The drawing under review shows one solid part. Ordinate dimensions are in mm from its lowest x, y, z. Coordinates: 2 decimals unless noted, no trailing zeros. Loops run counter-clockwise (first coordinate to the right, second up) from the corner with the lowest first, then second, coordinate; pieces in that order, holes last. Notation, with made-up numbers: (-20.75, 51.5) - (14.25, 51.5) arc R14 ccw to (14.25, 56.5) - close; hole circle Ø1 at (65.5, 43). An arc over 180 degrees is marked (long way). Answer as a JSON object with one key per item and string values. Group by question number.
Item 1: Mouldability with a two-part tool opening along Y and no side actions: class the marked faces 1, 2 and 3 as released by +Y, released by -Y, zero draft, split by the parting line, or undercut.
Item 2: Clearance check with flat-ended pins moving along their axes: pin 1 (6 mm diameter, centred on x = 5.5, y = 25, fed in from -Z); pin 2 (3 mm diameter, centred on y = 2.51, z = 2.5, fed in from -X); pin 3 (2 mm diameter, centred on y = 2.51, z = 2.5, fed in from -X). State where each tip first meets the part, or that it passes through.
Item 3: We need section D-D (y = 17). Give the boundary of the cut face in (x, z), then the cut area to 3 significant figures.
Item 4: We need section B-B (y = 13). Give the boundary of the cut face in (x, z).
Item 5: To check wall thickness, follow line 1 (X direction, y = 4.5, z = 4.55); line 2 (Y direction, x = 15.5, z = 1.55) (1 decimal); line 3 (X direction, y = 13, z = 3.5). State the ranges of each line that lie inside material, in increasing order.
Item 6: We need section C-C (x = 8.25). Give the boundary of the cut face in (y, z).
Item 7: We need section A-A (x = 16). Give the boundary of the cut face in (y, z).
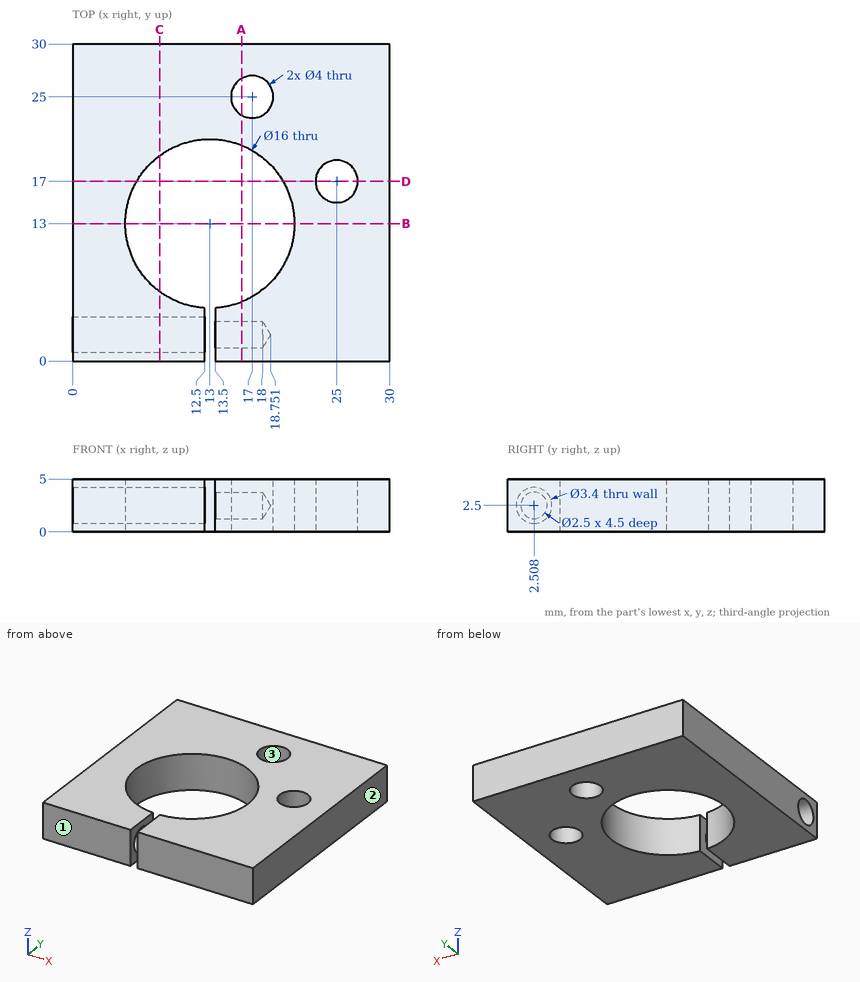
Check sheet entries:
{
 "1": {"face 1": "released by -Y", "face 2": "zero draft", "face 3": "undercut"},
 "2": {"pin 1": "stops at z = 0", "pin 2": "stops at x = 13.5", "pin 3": "stops at x = 18.15"},
 "3": {"outline": "(0, 0) - (6.07, 0) - (6.07, 5) - (0, 5) - close; (19.93, 0) - (23, 0) - (23, 5) - (19.93, 5) - close; (27, 0) - (30, 0) - (30, 5) - (27, 5) - close", "area": "60.7 mm2"},
 "4": {"outline": "(0, 0) - (5, 0) - (5, 5) - (0, 5) - close; (21, 0) - (30, 0) - (30, 5) - (21, 5) - close"},
 "5": {"line 1": "x = 0 to 12.5, 13.5 to 30", "line 2": "y = 0 to 1.7, 3.3 to 5.4, 20.6 to 23.7, 26.3 to 30", "line 3": "x = 0 to 5, 21 to 30"},
 "6": {"outline": "(0, 0) - (6.56, 0) - (6.56, 5) - (0, 5) - close; (19.44, 0) - (30, 0) - (30, 5) - (19.44, 5) - close; hole circle Ø3.4 at (2.51, 2.5)"},
 "7": {"outline": "(0, 0) - (5.58, 0) - (5.58, 5) - (0, 5) - close; (20.42, 0) - (23.27, 0) - (23.27, 5) - (20.42, 5) - close; (26.73, 0) - (30, 0) - (30, 5) - (26.73, 5) - close; hole circle Ø2.5 at (2.51, 2.5)"}
}
